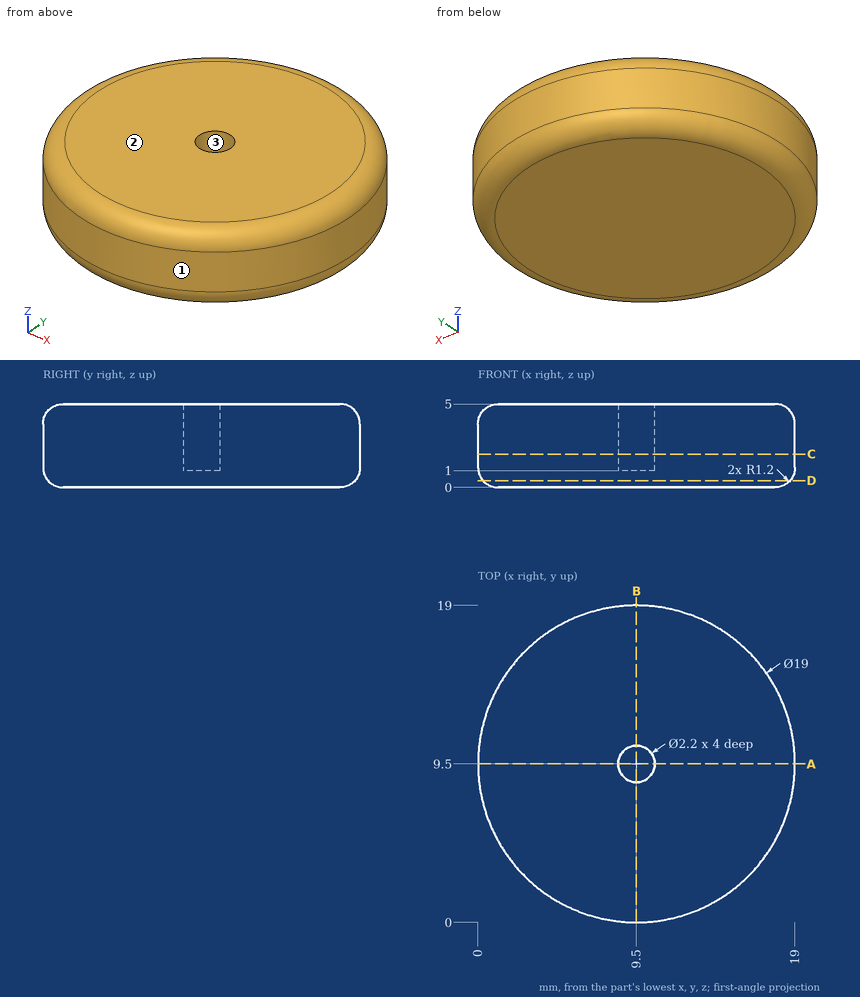
Geometry: see drawing. Coordinates: mm, zero at the bounding-box minimum. Round coordinates to 2 decimals unless told otherwise and drop trailing zeros. Loops run counter-clockwise (first coordinate to the right, second up) from the corner with the lowest first, then second, coordinate; pieces in that order, holes last. Notation, with made-up numbers: M -29,-24.75 L -11,-24.75 A22 cw -11,-9.75 Z; hole C 41.25,-11.5 d8. An arc over 180 degrees is marked long. Use a Markdown table: item, result. Add a question column.
1. Section query D-D on z = 0.4. Return the cut outline in (x, y).
2. Mould query, pull axis X, two halves, no side actions, for the marked faces 1, 2 and 3. Classes: pulls with the +X half, pulls with the -X half, needs draft (parallel to the pull), parting line crosses it, or undercut.
3. Contact query for flat-ended pins moving along their axis: P1, Ø2, axis at y = 12, z = 2, coming from the -X side; P2, Ø1, axis at y = 7, z = 1, coming from the -X side. Output: stop coordinate, or through.
4. Line query: line 1 (Y direction, x = 9.5, z = 2.4); line 2 (X direction, y = 9.25, z = 4.5); line 3 (Y direction, x = 11.5, z = 2.8). Output: solid intervals per line, ascending.
5. Section query C-C on z = 2. Return the cut outline in (x, y), then the cut area to 3 significant figures.
6. Section query A-A on y = 9.5. Return the cut outline in (x, z).
Reported:
| question | item | result |
|---|---|---|
| 1 | outline | C 9.5,9.5 d18.39 |
| 2 | face 1 | parting line crosses it |
| 2 | face 2 | needs draft |
| 2 | face 3 | undercut |
| 3 | P1 | stops at x = 0.12 |
| 3 | P2 | stops at x = 0.22 |
| 4 | line 1 | y = 0 to 8.4, 10.6 to 19 |
| 4 | line 2 | x = 0.23 to 8.43, 10.57 to 18.77 |
| 4 | line 3 | y = 0.21 to 18.79 |
| 5 | outline | C 9.5,9.5 d19; hole C 9.5,9.5 d2.2 |
| 5 | area | 280 mm² |
| 6 | outline | M 0,1.2 A1.2 ccw 1.2,0 L 17.8,0 A1.2 ccw 19,1.2 L 19,3.8 A1.2 ccw 17.8,5 L 10.6,5 L 10.6,1 L 8.4,1 L 8.4,5 L 1.2,5 A1.2 ccw 0,3.8 Z |
